Verification items for the finished model (mm, model axes). A direction names the side the tool comes from. Round coordinates to 2 decimals unless told otherwise and drop trailing zeros. Order: outer loops, then holes, each group sorted by start corner. A loop starts at its lowest first (then second) coordinate and runs counter-clockwise, first axis right, second up. Notation, with made-up numbers: (31.25, 78.5) -> (35.25, 78.5) arc R17 cw to (35.25, 108.5) -> close; hole circle Ø2 at (46.25, 52.25). An arc over 180 degrees is marked (long way). Put each result on its own line as item: value.
from build123d import *

# Parameters (mm, degrees)
F0_W      = 80
F0_H      = 110
F1_DEPTH  = 4.5
F2_W      = 10
F2_H      = 5
F3_DEPTH  = 4.501
F5_DEPTH  = 13.5
F6_R      = 3.8
F6_R_2    = 2.6
F7_DEPTH  = 4.501
F10_DEPTH = 13.5
F12_DEPTH = 3
F14_DEPTH = 3
F16_DEPTH = 3
F17_R     = 1.75
F18_DEPTH = 49.751
F19_R     = 1.75
F20_DEPTH = 76.9261442127
F21_R     = 1.75
F22_DEPTH = 76.9261442127
F24_DEPTH = 3
F25_R     = 1.5
F26_R     = 3
F27_R     = 2


with BuildPart() as f1:
    # F0 (on Top) → F1 (new body)
    with BuildSketch(Plane.XY):
        Rectangle(F0_W, F0_H)
    extrude(amount=F1_DEPTH)

    # F2 (on face) → F3 (cut, through all)
    with BuildSketch(Plane.XY.offset(4.5)):
        with Locations((0, 47.5)):
            Rectangle(F2_W, F2_H)
        with Locations((0, -47.5)):
            Rectangle(F2_W, F2_H)
    extrude(amount=-F3_DEPTH, mode=Mode.SUBTRACT)

    # F4 (on face) → F5 (join)
    with BuildSketch(Plane.XY.offset(4.5)):
        Polygon((40, 30.454058454), (0, -9.545941546), (-40, 30.454058454), (-40, 26.2114177669), (-9.75, -4.0385822331), (-9.75, -55), (-6.75, -55), (-6.75, -7.0385822331), (0, -13.7885822331), (6.75, -7.0385822331), (6.75, -55), (9.75, -55), (9.75, -4.0385822331), (40, 26.2114177669), align=None)
        Polygon((-40, 49.545941546), (0, 9.545941546), (40, 49.545941546), (40, 53.7885822331), (0, 13.7885822331), (-40, 53.7885822331), align=None)
    extrude(amount=F5_DEPTH)

    # F6 (on face) → F7 (cut, through all)
    with BuildSketch(Plane.XY.offset(4.5)):
        with Locations((21, -40)):
            Circle(F6_R)
        with Locations((21, 45)):
            Circle(F6_R)
        with Locations((-21, 45)):
            Circle(F6_R_2)
        with Locations((-21, -40)):
            Circle(F6_R_2)
    extrude(amount=-F7_DEPTH, mode=Mode.SUBTRACT)

    # F9 (on face) → F10 (join)
    with BuildSketch(Plane.XY.offset(18)):
        Polygon((-9.75, 23.5385822331), (-9.75, -55), (-6.75, -55), (-6.75, 20.5385822331), align=None)
        Polygon((9.75, 23.5385822331), (6.75, 20.5385822331), (6.75, -55), (9.75, -55), align=None)
    extrude(amount=F10_DEPTH)

    # F11 (on face) → F12 (join)
    with BuildSketch(Plane.XY.offset(18)):
        Polygon((9.75, 23.5385822331), (9.75, -4.0385822331), (40, 26.2114177669), (40, 53.7885822331), align=None)
        Polygon((-40, 53.7885822331), (-40, 26.2114177669), (-9.75, -4.0385822331), (-9.75, 23.5385822331), align=None)
    extrude(amount=F12_DEPTH)

    # F13 (on offset) → F14 (join)
    with BuildSketch(Plane.XY.offset(18)):
        Polygon((0, -13.7885822331), (-6.75, -7.0385822331), (-6.75, -55), (6.75, -55), (6.75, -7.0385822331), align=None)
    extrude(amount=-F14_DEPTH)

    # F15 (on face) → F16 (join)
    with BuildSketch(Plane.XY.offset(31.5)):
        Polygon((-9.75, 23.5385822331), (-9.75, -55), (9.75, -55), (9.75, 23.5385822331), (0, 13.7885822331), align=None)
    extrude(amount=F16_DEPTH)

    # F17 (on face) → F18 (cut, through all)
    with BuildSketch(Plane.YZ.offset(9.75)):
        with Locations((-15, 24.75)):
            Circle(F17_R)
    extrude(amount=-F18_DEPTH, mode=Mode.SUBTRACT)

    # F19 (on face) → F20 (cut, through all)
    with BuildSketch(Plane(origin=(6.8942911166, -6.8942911166, 0), x_dir=(0.7071067812, 0.7071067812, 0), z_dir=(0.7071067812, -0.7071067812, 0))):
        with Locations((26.8185424949, 11.25)):
            Circle(F19_R)
    extrude(amount=-F20_DEPTH, mode=Mode.SUBTRACT)

    # F21 (on face) → F22 (cut, through all)
    with BuildSketch(Plane(origin=(-6.8942911166, -6.8942911166, 0), x_dir=(0.7071067812, -0.7071067812, 0), z_dir=(-0.7071067812, -0.7071067812, 0))):
        with Locations((-26.8185424949, 11.25)):
            Circle(F21_R)
    extrude(amount=-F22_DEPTH, mode=Mode.SUBTRACT)

    # F23 (on face) → F24 (join)
    with BuildSketch(Plane.XZ.offset(55)):
        Polygon((40, 4.5), (9.75, 34.5), (9.75, 4.5), align=None)
        Polygon((-40, 4.5), (-9.75, 4.5), (-9.75, 34.5), align=None)
    extrude(amount=-F24_DEPTH)

    # F25
    f25_edges = [f1.edges().sort_by_distance(p)[0] for p in [
        (0, 50, 4.5),
        (0, 50, 0),
        (0, -50, 0),
        (0, -50, 4.5),
    ]]
    fillet(f25_edges, radius=F25_R)

    # F26
    f26_edges = [f1.edges().sort_by_distance(p)[0] for p in [
        (-9.75, -52, 19.5),
        (-9.75, 9.75, 21),
        (-9.75, -28.019291, 4.5),
        (-24.875, -52, 4.5),
        (-9.75, -4.038582, 12.75),
        (-24.875, 11.086418, 4.5),
        (24.875, -52, 4.5),
        (9.75, -52, 19.5),
        (9.75, -28.019291, 4.5),
        (9.75, -4.038582, 12.75),
        (9.75, 9.75, 21),
        (24.875, 11.086418, 4.5),
    ]]
    fillet(f26_edges, radius=F26_R)

    # F27
    f27_edges = [f1.edges().sort_by_distance(p)[0] for p in [
        (-40, 55, 2.25),
        (40, 55, 2.25),
    ]]
    fillet(f27_edges, radius=F27_R)


solid = f1.part
Item 1: Section check C-C on x = -3. State how many separate pieces and enclosed holes the cut face has, then the cut area to 3 significant figures.
Check sheet entries:
separate pieces: 4
enclosed holes: 0
area: 911 mm^2
Item 2: Release check for a two-part mould opening along Y. For faces 6 (the cylindrical face through (-10.65, 10.85, 21.86)), 7 (the cylindrical face through (-10.65, -27.45, 5.36)), 8 (the flat face through (-19.66, 33.45, 12.62)) record: +Y half, -Y half, draft (parallel to the pull), parting line (faces both ways), or undercut.
Check sheet entries:
face 6: draft
face 7: undercut
face 8: +Y half
Item 3: Section check B-B on y = -40. Record the boundary of the cut face in (x, z), then the cut area to 3 significant figures.
Check sheet entries:
outline: (-40, 0) -> (-23.6, 0) -> (-23.6, 4.5) -> (-40, 4.5) -> close; (-18.4, 0) -> (17.2, 0) -> (17.2, 4.5) -> (12.75, 4.5) arc R3 cw to (9.75, 7.5) -> (9.75, 34.5) -> (-9.75, 34.5) -> (-9.75, 7.5) arc R3 cw to (-12.75, 4.5) -> (-18.4, 4.5) -> close; (24.8, 0) -> (40, 0) -> (40, 4.5) -> (24.8, 4.5) -> close; hole (-6.75, 4.5) -> (6.75, 4.5) -> (6.75, 15) -> (-6.75, 15) -> close; hole (-6.75, 18) -> (6.75, 18) -> (6.75, 31.5) -> (-6.75, 31.5) -> close
area: 567 mm^2
Item 4: Material ranges on L1, parallel to Y at x = 21, z = 2.7; L2, parallel to Z at x = -4, y = -30; L3, parallel to Y at x = -21, z = 3.1, recorded low to high. Write a range as [from, to].
Check sheet entries:
L1: y = [-55, -43.8], [-36.2, 41.2], [48.8, 55]
L2: z = [0, 4.5], [15, 18], [31.5, 34.5]
L3: y = [-55, -42.6], [-37.4, 42.4], [47.6, 55]
Item 5: Gauge pin test, flat ends, axial feed: pin 1 Ø8 at (y, z) = (14, 12) entering from -X; pin 2 Ø3 at (x, y) = (-21, 45) entering from +Z; pin 3 Ø4 at (y, z) = (-15, 24.75) entering from +X; pin 4 Ø4 at (y, z) = (0, 28) entering from -X. Record the tip position at first contact, or that the pin passes through.
Check sheet entries:
pin 1: stops at x = -31.79
pin 2: passes through
pin 3: stops at x = 9.75
pin 4: stops at x = -9.75
Item 6: Tool access check on faces 1 (the flat face through (-27, 27, 21)), 2 (the flat face through (25.11, 11.32, 14.59)), 3 (the cylindrical face through (-9.985, -4.118, 15.634)), 4 (the cylindrical face through (10.65, 10.41, 21.86)), 5 (the flat face through (25.087, -53.375, 19.29)). Record the directions out of +Z, -Z, +X, -X, +Y, -Y that give a thin tool (end or side, any length) a straight path to the whole face; none if there is none.
Check sheet entries:
face 1: +Z, -X, +Y
face 2: +Z, +X
face 3: +Z, -X
face 4: +Z, +X, +Y
face 5: +Z, +X, -Y
Item 7: Section check A-A on y = -15. Record the boundary of the cut face in (x, z).
Check sheet entries:
outline: (-40, 0) -> (40, 0) -> (40, 4.5) -> (12.75, 4.5) arc R3 cw to (9.75, 7.5) -> (9.75, 23) -> (6.75, 23) -> (6.75, 18) -> (-6.75, 18) -> (-6.75, 23) -> (-9.75, 23) -> (-9.75, 7.5) arc R3 cw to (-12.75, 4.5) -> (-40, 4.5) -> close; (-9.75, 26.5) -> (-6.75, 26.5) -> (-6.75, 31.5) -> (6.75, 31.5) -> (6.75, 26.5) -> (9.75, 26.5) -> (9.75, 34.5) -> (-9.75, 34.5) -> close; hole (-6.75, 4.5) -> (6.75, 4.5) -> (6.75, 15) -> (-6.75, 15) -> close
